For this review, take the finished solid that the model builds, in its own axes (mm). A direction names the side the tool comes from. Coordinates: 2 decimals unless noted, no trailing zeros. Write each loop counter-clockwise with the first axis right and the second up, starting at its lowest first coordinate (ties: lowest second). Pieces come first, ordered by that corner, then holes. Notation, with made-up numbers: M 1,34 L 47,34 A7 ccw 47,42 Z; hole C -35.75,17 d7. An arc over 180 degrees is marked long. Return JSON: item names as keys, results as strings.
```python
from build123d import *

# Parameters (mm, degrees)
BOSS_EXTRUDE2_DEPTH     = 15.24
SKETCH5_R               = 7.62
CUT_EXTRUDE2_DEPTH      = 15.24
BOSS_EXTRUDE3_DEPTH     = 2.54
CUT_EXTRUDE5_DEPTH      = 41.652633663
CUT_EXTRUDE5_DEPTH_BACK = 41.652633663
SKETCH7_R               = 1.0033


with BuildPart() as part:
    # Sketch1 → Boss-Extrude2 (new body)
    with BuildSketch(Plane.XY):
        with BuildLine():
            Line((-17.763499893, 14.683044609), (-17.763499893, -17.608986031))
            Line((-17.763499893, -17.608986031), (-10.024087591, -22.679635471))
            Line((-10.024087591, -22.679635471), (-10.024087591, -19.359490178))
            Line((-10.024087591, -19.359490178), (10.024087591, -19.359490178))
            Line((10.024087591, -19.359490178), (10.024087591, -22.679635471))
            Line((10.024087591, -22.679635471), (17.763499893, -17.608986031))
            Line((17.763499893, -17.608986031), (17.763499893, 14.683044609))
            ThreePointArc((17.763499893, 14.683044609), (12.2054587, 19.511759091), (5.051122326, 21.250660037))
            Line((5.051122326, 21.250660037), (5.051122326, 19.699745061))
            Line((5.051122326, 19.699745061), (-5.051122326, 19.699745061))
            Line((-5.051122326, 19.699745061), (-5.051122326, 21.250660037))
            ThreePointArc((-5.051122326, 21.250660037), (-12.2054587, 19.511759091), (-17.763499893, 14.683044609))
        make_face()
    extrude(amount=BOSS_EXTRUDE2_DEPTH)

    # Sketch5 → Cut-Extrude2 (cut)
    with BuildSketch(Plane.XY.offset(15.24)):
        Circle(SKETCH5_R)
    extrude(amount=-CUT_EXTRUDE2_DEPTH, mode=Mode.SUBTRACT)

    # Sketch6 → Boss-Extrude3 (add)
    with BuildSketch(Plane.XY.offset(15.24)):
        with BuildLine():
            Line((-27.497120647, 3.03730764), (-17.763499893, 5.900096548))
            Line((-17.763499893, 5.900096548), (-17.763499893, -5.920973667))
            Line((-17.763499893, -5.920973667), (-27.497120647, -3.058184758))
            ThreePointArc((-27.497120647, -3.058184758), (-29.216566103, -1.891287663), (-30.10005247, -0.010438559))
            ThreePointArc((-30.10005247, -0.010438559), (-29.216566103, 1.870410544), (-27.497120647, 3.03730764))
        make_face()
        with BuildLine():
            Line((27.497120647, 3.03730764), (17.763499893, 5.900096548))
            Line((17.763499893, 5.900096548), (17.763499893, -5.920973667))
            Line((17.763499893, -5.920973667), (27.497120647, -3.058184758))
            ThreePointArc((27.497120647, -3.058184758), (29.216566103, -1.891287663), (30.10005247, -0.010438559))
            ThreePointArc((30.10005247, -0.010438559), (29.216566103, 1.870410544), (27.497120647, 3.03730764))
        make_face()
    extrude(amount=-BOSS_EXTRUDE3_DEPTH)

    # Sketch7 → Cut-Extrude5 (cut, two sides: drawn at the far end of the back side and taken through both)
    with BuildSketch(Plane(origin=(0, 0, 0), x_dir=(-1, 0, 0), z_dir=(0, 0, -1)).offset(-CUT_EXTRUDE5_DEPTH_BACK)):
        with Locations(Location((-19.685, 0, 0), (0, 0, 180))):
            Circle(SKETCH7_R)
        with Locations(Location((-26.416, 0, 0), (0, 0, 180))):
            Circle(SKETCH7_R)
        with Locations(Location((19.685, 0, 0), (0, 0, 180))):
            Circle(SKETCH7_R)
        with Locations(Location((26.416, 0, 0), (0, 0, 180))):
            Circle(SKETCH7_R)
    extrude(amount=CUT_EXTRUDE5_DEPTH + CUT_EXTRUDE5_DEPTH_BACK, mode=Mode.SUBTRACT)


solid = part.part
```
1. Clearance check with flat-ended pins moving along their axes: pin 1 Ø0.8 at (y, z) = (20.5, 10.5) entering from +X; pin 2 Ø3 at (x, z) = (-1.5, 6) entering from +Y; pin 3 Ø4 at (y, z) = (-12, 9.5) entering from -X. State where each tip first meets the part, or that it passes through.
Checks:
{"pin 1": "x = 10.93", "pin 2": "y = 19.7", "pin 3": "x = -17.76"}
2. For faces 4 (the face through (10.024, -21, 8)), 5 (the face through (-22, 0, 12.7)), 6 (the face through (22, 0, 12.7)), list the 3-axis set-ups (+Z, -Z, +X, -X, +Y, -Y) from which the entire face can be reached by the end or side of a thin tool; tool diameter is ignored.
Checks:
{"face 4": "+Z, -Z, -Y", "face 5": "-Z, -X, +Y, -Y", "face 6": "-Z, +X, +Y, -Y"}
3. We need section C-C (y = 2). State the section outline as (x, z) points.
Checks:
{"outline": "M -29.1,12.7 L -17.76,12.7 L -17.76,0 L -7.35,0 L -7.35,15.24 L -29.1,15.24 Z; M 7.35,0 L 17.76,0 L 17.76,12.7 L 29.1,12.7 L 29.1,15.24 L 7.35,15.24 Z"}
4. We need section D-D (z = 14.25). State the section outline as (x, y) points (1 decimal), plus the area to 3 significant figures.
Checks:
{"outline": "M -30.1,0 A3.9 ccw -27.5,-3.1 L -17.8,-5.9 L -17.8,-17.6 L -10,-22.7 L -10,-19.4 L 10,-19.4 L 10,-22.7 L 17.8,-17.6 L 17.8,-5.9 L 27.5,-3.1 A3.9 ccw 30.1,0 A3.9 ccw 27.5,3 L 17.8,5.9 L 17.8,14.7 A15.6 ccw 5.1,21.3 L 5.1,19.7 L -5.1,19.7 L -5.1,21.3 A15.6 ccw -17.8,14.7 L -17.8,5.9 L -27.5,3 A3.9 ccw Z; hole C -26.4,0 d2; hole C -19.7,0 d2; hole C 0,0 d15.2; hole C 19.7,0 d2; hole C 26.4,0 d2", "area": "1,390 mm2"}
5. We need section A-A (x = 0). State the section outline as (y, z) points, plus the area to 3 significant figures.
Checks:
{"outline": "M -19.36,0 L -7.62,0 L -7.62,15.24 L -19.36,15.24 Z; M 7.62,0 L 19.7,0 L 19.7,15.24 L 7.62,15.24 Z", "area": "363 mm2"}
6. Draft analysis for pull direction Y (two halves, no side actions). For faces 1 (the face through (-1.65, -7.44, 7.73)), 2 (the face through (29.2, -1.91, 13.99)), 3 (the face through (-5.051, 20, 8)), state which applies: +Y half, -Y half, draft (parallel to the pull), parting line (faces both ways), or undercut.
Checks:
{"face 1": "undercut", "face 2": "-Y half", "face 3": "draft"}
7. We need section B-B (z = 7.5). State the section outline as (x, y) points, plus the area to 3 significant figures.
Checks:
{"outline": "M -17.76,-17.61 L -10.02,-22.68 L -10.02,-19.36 L 10.02,-19.36 L 10.02,-22.68 L 17.76,-17.61 L 17.76,14.68 A15.59 ccw 5.05,21.25 L 5.05,19.7 L -5.05,19.7 L -5.05,21.25 A15.59 ccw -17.76,14.68 Z; hole C 0,0 d15.24", "area": "1,210 mm2"}
8. Wall thickness on L1, parallel to Z at x = -19.5, y = 4; L2, parallel to X at y = -15, z = 14; L3, parallel to X at y = 6, z = 0.5: over which ranges is each line inside the solid? List them lowest first. Write a range as from..to.
Checks:
{"L1": "12.7..15.24", "L2": "-17.76..17.76", "L3": "-17.76..-4.7, 4.7..17.76"}
